```python
from build123d import *

# Parameters (mm, degrees)
EXTRUDE_1_DEPTH     = 83
CUT_EXTRUDE_START   = -10
SKETCH_6_R          = 1.6
CUT_EXTRUDE_1_DEPTH = 15
SKETCH_5_R          = 3.5
CUT_EXTRUDE_2_DEPTH = 2


with BuildPart() as part:
    # 草图1 → 凸台-拉伸1 (new body)
    with BuildSketch(Plane.XY):
        with BuildLine():
            Line((0, 0), (10, 0))
            Line((10, 0), (10, 5))
            ThreePointArc((10, 5), (5, 5.250628145), (0, 5))
            Line((0, 5), (0, 0))
        make_face()
    extrude(amount=EXTRUDE_1_DEPTH)

    # 草图6 → 切除-拉伸1 (cut)
    with BuildSketch(Plane(origin=(0, 5, 0), x_dir=(1, 0, 0), z_dir=(0, 1, 0)).offset(CUT_EXTRUDE_START)):
        with Locations((5, -71.5)):
            Circle(SKETCH_6_R)
    cut_extrude_1 = extrude(amount=CUT_EXTRUDE_1_DEPTH, mode=Mode.SUBTRACT)

    # 草图5 → 切除-拉伸2 (cut, symmetric)
    with BuildSketch(Plane(origin=(0, 5, 0), x_dir=(1, 0, 0), z_dir=(0, 1, 0))):
        with Locations((5, -71.5)):
            Circle(SKETCH_5_R)
    cut_extrude_2 = extrude(amount=CUT_EXTRUDE_2_DEPTH, both=True, mode=Mode.SUBTRACT)

    # 镜向1: 切除-拉伸1, 切除-拉伸2 across plane
    add(cut_extrude_1.mirror(Plane(origin=(0, 0, 41.5), x_dir=(1, 0, 0), z_dir=(0, 0, -1))), mode=Mode.SUBTRACT)
    add(cut_extrude_2.mirror(Plane(origin=(0, 0, 41.5), x_dir=(1, 0, 0), z_dir=(0, 0, -1))), mode=Mode.SUBTRACT)


solid = part.part
```
The listing builds one solid part. Answer for the finished solid, in the listing's coordinates (mm). A direction names the side the tool comes from. Round coordinates to 2 decimals unless told otherwise and drop trailing zeros. Write each loop counter-clockwise with the first axis right and the second up, starting at its lowest first coordinate (ties: lowest second). Pieces come first, ordered by that corner, then holes. Notation, with made-up numbers: (45.25, 83) -> (57.25, 83) arc R26 cw to (57.25, 98) -> close; hole circle Ø2 at (45.5, 62). An arc over 180 degrees is marked (long way). Write item = value, one per line.
1) Given pin 1 (5 mm diameter, centred on x = 1, z = 12.5, fed in from +Y), flat-ended and moving along its own axis, determine where the tip first touches the part or whether it passes through.
Check values:
pin_1 = 5.2
2) Which of the six approach directions +Z, -Z, +X, -X, +Y, -Y give full straight-line access (tool end or side, diameter ignored) to faces 1 (the cylindrical face through (6.615, 4.143, 8.395)), 2 (the flat face through (5, 3, 83))?
Check values:
face_1 = +Y
face_2 = +Z, +X, -X, +Y, -Y
3) Section A-A on y = 3.8 is taken. Write down the section's boundary in (x, z).
Check values:
outline = (0, 0) -> (10, 0) -> (10, 83) -> (0, 83) -> close; hole circle Ø7 at (5, 11.5); hole circle Ø7 at (5, 71.5)
4) Section B-B on z = 11.5 is taken. Write down the section's boundary in (x, y), plus the area to 3 significant figures.
Check values:
outline = (0, 0) -> (3.4, 0) -> (3.4, 3) -> (1.5, 3) -> (1.5, 5.13) arc R50 ccw to (0, 5) -> close; (6.6, 0) -> (10, 0) -> (10, 5) arc R50 ccw to (8.5, 5.13) -> (8.5, 3) -> (6.6, 3) -> close
area = 26.6 mm²
5) Straight lines are drawn through the part: line 1 along Z through (x, y) = (5, 0.95); line 2 along Z through (x, y) = (5, 4.3); line 3 along X through (y, z) = (2, 71.5). For each, find the intervals that lie inside material, in ascending order. Write a range as [from, to].
Check values:
line_1 = [0, 9.9], [13.1, 69.9], [73.1, 83]
line_2 = [0, 8], [15, 68], [75, 83]
line_3 = [0, 3.4], [6.6, 10]
6) Section D-D on z = 33 is taken. Write down the section's boundary in (x, y).
Check values:
outline = (0, 0) -> (10, 0) -> (10, 5) arc R50 ccw to (0, 5) -> close
7) Section C-C on x = 7.5 is taken. Write down the section's boundary in (y, z).
Check values:
outline = (0, 0) -> (5.19, 0) -> (5.19, 9.05) -> (3, 9.05) -> (3, 13.95) -> (5.19, 13.95) -> (5.19, 69.05) -> (3, 69.05) -> (3, 73.95) -> (5.19, 73.95) -> (5.19, 83) -> (0, 83) -> close
